Read the model definition and answer for the solid it produces. Units are mm, in the model's axes. Coordinates: 2 decimals unless noted, no trailing zeros. Loops run counter-clockwise (first coordinate to the right, second up) from the corner with the lowest first, then second, coordinate; pieces in that order, holes last. Notation, with made-up numbers: M -7.5,-12 L 37.5,-12 A24 cw 37.5,26 Z; hole C 56.5,41 d3. An arc over 180 degrees is marked long. One line per item, written item: value. Start each with the question number.
1. A flat-ended cylindrical pin translates along its axis: pin 1 (13 mm diameter, centred on x = 0, y = -15.99, fed in from -Z). Find the tip coordinate at first contact, or state that the pin passes through.
2. Consider probe 1 along Y at (x, z) = (3.5, 1.5); probe 2 along Y at (x, z) = (-2.5, 0.5); probe 3 along X at (y, z) = (-12.5, 0.4). Determine where each line is inside the solid, lowest interval first.
3. The part is cut by section C-C (x = -8.5). Write down the section's boundary in (y, z), then the cut area to 3 significant figures.
4. The part is cut by section B-B (y = -24). Write down the section's boundary in (x, z).
5. The part is cut by section A-A (z = 1). Write down the section's boundary in (x, y) (3 decimals), then the cut area to 3 significant figures.
```python
from build123d import *

# Parameters (mm, degrees)
F0_R     = 3.995
F1_DEPTH = 2
F2_DEPTH = 25


with BuildPart() as f1:
    # F0 (on Top) → F1 (new body)
    with BuildSketch(Plane.XY):
        with BuildLine():
            Line((-13.49, -29.49), (13.49, -29.49))
            Line((13.49, -29.49), (13.49, -15.9924751222))
            ThreePointArc((13.49, -15.9924751222), (0, -29.4824751222), (-13.49, -15.9924751222))
            Line((-13.49, -15.9924751222), (-13.49, -29.49))
        make_face()
        with BuildLine():
            ThreePointArc((2.8439841916, -2.8056690678), (10.4963195156, -7.5185517908), (13.49, -15.9924751222))
            Line((13.49, -15.9924751222), (13.49, 16))
            ThreePointArc((13.49, 16), (10.4943486529, 7.5236360182), (2.8378508003, 2.8118726562))
            ThreePointArc((2.8378508003, 2.8118726563), (3.6944038049, 1.5203307293), (3.995, 0))
            ThreePointArc((3.995, 0), (3.6960615421, -1.5162961707), (2.8439841916, -2.8056690678))
        make_face()
        with BuildLine():
            ThreePointArc((-13.49, -15.9924751222), (0, -29.4824751222), (13.49, -15.9924751222))
            ThreePointArc((13.49, -15.9924751222), (10.4963195156, -7.5185517908), (2.8439841916, -2.8056690678))
            ThreePointArc((2.8439841916, -2.8056690678), (0, -3.995), (-2.8439841916, -2.8056690678))
            ThreePointArc((-2.8439841916, -2.8056690678), (-10.4963195156, -7.5185517908), (-13.49, -15.9924751222))
        make_face()
        with Locations((0, -15.9924751222)):
            Circle(F0_R, mode=Mode.SUBTRACT)
        with BuildLine():
            Line((-13.49, 16.000000062), (-13.49, -15.9924751222))
            ThreePointArc((-13.49, -15.9924751222), (-10.4963195156, -7.5185517908), (-2.8439841916, -2.8056690678))
            ThreePointArc((-2.8439841916, -2.8056690678), (-3.9949976188, 0.0043618516), (-2.8378508003, 2.8118726563))
            ThreePointArc((-2.8378508003, 2.8118726562), (-10.4943486724, 7.5236360423), (-13.49, 16.000000062))
        make_face()
        with BuildLine():
            ThreePointArc((0, 29.49), (9.5388704782, 25.5388704782), (13.49, 16))
            Line((13.49, 16), (13.49, 29.49))
            Line((13.49, 29.49), (0, 29.49))
        make_face()
        with BuildLine():
            ThreePointArc((2.8378508003, 2.8118726562), (10.4943486529, 7.5236360182), (13.49, 16))
            ThreePointArc((13.49, 16), (9.5388704782, 25.5388704782), (0, 29.49))
            ThreePointArc((0, 29.49), (-9.5388704563, 25.5388705001), (-13.49, 16.000000062))
            ThreePointArc((-13.49, 16.000000062), (-10.4943486724, 7.5236360423), (-2.8378508003, 2.8118726562))
            ThreePointArc((-2.8378508003, 2.8118726563), (0, 3.995), (2.8378508003, 2.8118726563))
        make_face()
        with Locations((0, 16)):
            Circle(F0_R, mode=Mode.SUBTRACT)
        with BuildLine():
            Line((-13.49, 29.49), (-13.49, 16.000000062))
            ThreePointArc((-13.49, 16.000000062), (-9.5388704563, 25.5388705001), (0, 29.49))
            Line((0, 29.49), (-13.49, 29.49))
        make_face()
    extrude(amount=F1_DEPTH)

    # F0 (on Top) → F2 (cut)
    with BuildSketch(Plane.XY):
        with BuildLine():
            ThreePointArc((0, 29.49), (9.5388704782, 25.5388704782), (13.49, 16))
            Line((13.49, 16), (13.49, 29.49))
            Line((13.49, 29.49), (0, 29.49))
        make_face()
        with BuildLine():
            Line((-13.49, -29.49), (13.49, -29.49))
            Line((13.49, -29.49), (13.49, -15.9924751222))
            ThreePointArc((13.49, -15.9924751222), (0, -29.4824751222), (-13.49, -15.9924751222))
            Line((-13.49, -15.9924751222), (-13.49, -29.49))
        make_face()
        with BuildLine():
            Line((-13.49, 29.49), (-13.49, 16.000000062))
            ThreePointArc((-13.49, 16.000000062), (-9.5388704563, 25.5388705001), (0, 29.49))
            Line((0, 29.49), (-13.49, 29.49))
        make_face()
    extrude(amount=F2_DEPTH, mode=Mode.SUBTRACT)


solid = f1.part
```
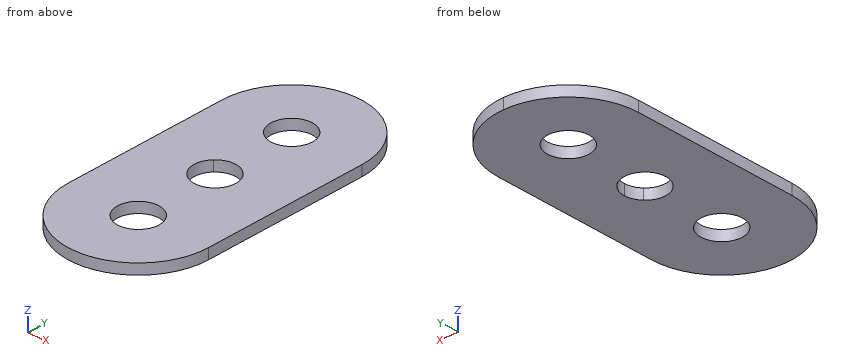
Answer block:
1. pin 1: stops at z = 0
2. probe 1: y = -29.02 to -17.92, -14.07 to -1.93, 1.93 to 14.07, 17.93 to 29.03
2. probe 2: y = -29.25 to -19.11, -12.88 to -3.12, 3.12 to 12.88, 19.12 to 29.26
2. probe 3: x = -13.49 to -1.94, 1.94 to 13.49
3. outline: M -26.47,0 L 26.48,0 L 26.48,2 L -26.47,2 Z
3. area: 106 mm2
4. outline: M -10.86,0 L 10.86,0 L 10.86,2 L -10.86,2 Z
5. outline: M -13.49,-15.992 A13.49 ccw 13.49,-15.992 L 13.49,16 A13.49 ccw -13.49,16 Z; hole C 0,-15.992 d7.99; hole C 0,0 d7.99; hole C 0,16 d7.99
5. area: 1,280 mm2
